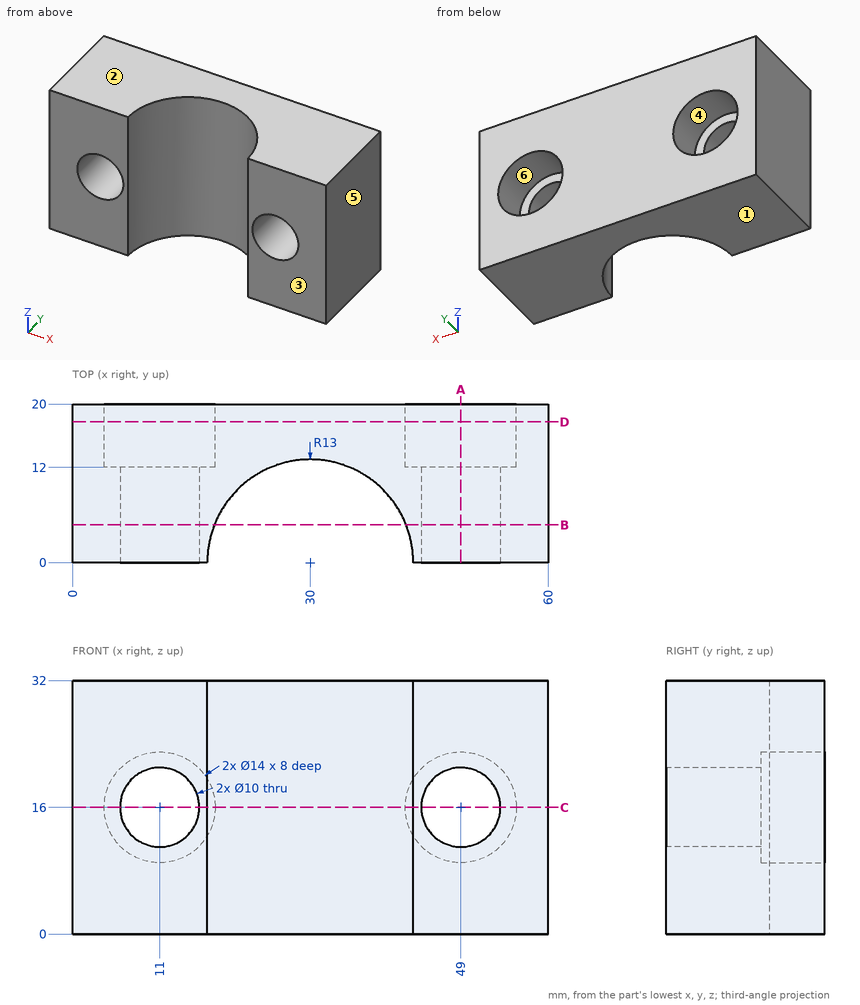
Here's the drawing with two shaded views (mm, measured from the low corner). I have some questions. A direction names the side the tool comes from. Give positions to 0.01 mm unless a question says otherwise; leave off trailing zeros. Loops run counter-clockwise (first coordinate to the right, second up) from the corner with the lowest first, then second, coordinate; pieces in that order, holes last. Notation, with made-up numbers: (3.5, 71) - (23.5, 71) arc R23 ccw to (23.5, 105) - close; hole circle Ø5 at (-5.75, 75). An arc over 180 degrees is marked (long way). Answer in a Markdown table with one row per item. Add a question column.
Q1. Which directions (+Z, -Z, +X, -X, +Y, -Y) give clear straight access to the entire face, cutting with the end or side of a thin tool? Please do the marked faces 5 and 6.
Q2. For pin 1 (8 mm diameter, centred on x = 33.5, z = 13.5, fed in from -Y); pin 2 (11 mm diameter, centred on x = 49.5, z = 17, fed in from +Y), each with a flat end and sliding along its axis, tell me the tip position at first contact or that it passes through.
Q3. We'd pull the mould along Z, two halves only. Please class the marked faces 1, 2, 3 and 4: +Z half, -Z half, draft (parallel to the pull), parting line (faces both ways), or undercut.
Q4. If we section it at D-D (y = 17.75): List the corners of the cut face in (x, z) for me.
Q5. If we section it at C-C (z = 16): List the corners of the cut face in (x, y) for me.
Q6. If we section it at B-B (y = 4.75): List the corners of the cut face in (x, z) for me.
Q7. Please list where these lines run through material, in increasing order: L1, parallel to X at y = 15, z = 16; L2, parallel to Z at x = 49, y = 14.5; L3, parallel to X at y = 9, z = 16. Write a range as from..to.
Q8. If we section it at A-A (x = 49): List the corners of the cut face in (y, z) for me.
The answers:
| question | item | result |
|---|---|---|
| 1 | face 5 | +Z, -Z, +X, +Y, -Y |
| 1 | face 6 | +Y |
| 2 | pin 1 | stops at y = 10.62 |
| 2 | pin 2 | stops at y = 12 |
| 3 | face 1 | -Z half |
| 3 | face 2 | +Z half |
| 3 | face 3 | draft |
| 3 | face 4 | undercut |
| 4 | outline | (0, 0) - (60, 0) - (60, 32) - (0, 32) - close; hole circle Ø14 at (11, 16); hole circle Ø14 at (49, 16) |
| 5 | outline | (0, 0) - (6, 0) - (6, 12) - (4, 12) - (4, 20) - (0, 20) - close; (16, 0) - (17, 0) arc R13 cw to (43, 0) - (44, 0) - (44, 12) - (42, 12) - (42, 20) - (18, 20) - (18, 12) - (16, 12) - close; (54, 0) - (60, 0) - (60, 20) - (56, 20) - (56, 12) - (54, 12) - close |
| 6 | outline | (0, 0) - (17.9, 0) - (17.9, 32) - (0, 32) - close; (42.1, 0) - (60, 0) - (60, 32) - (42.1, 32) - close; hole circle Ø10 at (11, 16); hole circle Ø10 at (49, 16) |
| 7 | L1 | x = 0..4, 18..42, 56..60 |
| 7 | L2 | z = 0..9, 23..32 |
| 7 | L3 | x = 0..6, 16..20.62, 39.38..44, 54..60 |
| 8 | outline | (0, 0) - (20, 0) - (20, 9) - (12, 9) - (12, 11) - (0, 11) - close; (0, 21) - (12, 21) - (12, 23) - (20, 23) - (20, 32) - (0, 32) - close |
